```python
from build123d import *

# Parameters (mm, degrees)
BOSS_EXTRUDE1_DEPTH = 12
SKETCH3_R           = 2
CUT_EXTRUDE1_DEPTH  = 10
SKETCH4_R           = 3
CUT_EXTRUDE2_DEPTH  = 10


with BuildPart() as part:
    # Sketch2 → Boss-Extrude1 (new body)
    with BuildSketch(Plane.XY):
        with BuildLine():
            Line((-25, 0), (-12.5, 0))
            ThreePointArc((-12.5, 0), (0, 12.5), (12.5, 0))
            Line((12.5, 0), (25, 0))
            ThreePointArc((25, 0), (24.873403825, 2.51272405), (24.494897428, 5))
            Line((24.494897428, 5), (21.563858653, 5))
            ThreePointArc((21.563858653, 5), (19.850737931, 5.537233793), (18.751181437, 6.956521739))
            ThreePointArc((18.751181437, 6.956521739), (0, 20), (-18.751181437, 6.956521739))
            ThreePointArc((-18.751181437, 6.956521739), (-19.850737931, 5.537233793), (-21.563858653, 5))
            Line((-21.563858653, 5), (-24.494897428, 5))
            ThreePointArc((-24.494897428, 5), (-24.873403825, 2.51272405), (-25, 0))
        make_face()
    extrude(amount=BOSS_EXTRUDE1_DEPTH)

    # Sketch3 → Cut-Extrude1 (cut)
    with BuildSketch(Plane(origin=(0, 0, 0), x_dir=(1, 0, 0), z_dir=(0, 1, 0))):
        with Locations(Location((20, -6, 0), (0, 0, 128.638810709))):
            Circle(SKETCH3_R)
        with Locations(Location((-20, -6, 0), (0, 0, 90))):
            Circle(SKETCH3_R)
    extrude(amount=CUT_EXTRUDE1_DEPTH, mode=Mode.SUBTRACT)

    # Sketch4 → Cut-Extrude2 (cut)
    with BuildSketch(Plane(origin=(0, 5, 0), x_dir=(1, 0, 0), z_dir=(0, 1, 0))):
        with Locations((20, -6)):
            Circle(SKETCH4_R)
        with Locations((-20, -6)):
            Circle(SKETCH4_R)
    extrude(amount=CUT_EXTRUDE2_DEPTH, mode=Mode.SUBTRACT)


solid = part.part
```
Input: part model. Units: mm. Frame: model coordinates. Give positions to 0.01 mm unless a question says otherwise; leave off trailing zeros. Order: outer loops, then holes, each group sorted by start corner. A loop starts at its lowest first (then second) coordinate and runs counter-clockwise, first axis right, second up. Notation, with made-up numbers: (-28.5, 33.5) - (28.5, 33.5) arc R5 cw to (28.5, 41.5) - close; hole circle Ø6 at (-22, -38). An arc over 180 degrees is marked (long way). Put each result on its own line as item: value.
Item 1: Section query A-A, the plane z = 6. Return loops of the section in (x, y), then the cut area to 3 significant figures.
Found:
outline: (-25, 0) - (-22, 0) - (-22, 5) - (-24.49, 5) arc R25 ccw to start; (-18, 0) - (-12.5, 0) arc R12.5 cw to (12.5, 0) - (18, 0) - (18, 5) - (17, 5) - (17, 10.54) arc R20 ccw to (-17, 10.54) - (-17, 5) - (-18, 5) - close; (22, 0) - (25, 0) arc R25 ccw to (24.49, 5) - (22, 5) - close
area: 378 mm^2
Item 2: Section query B-B, the plane x = -20. Return loops of the section in (y, z), then the cut area to 3 significant figures.
Found:
outline: (0, 0) - (5.44, 0) - (5.44, 3) - (5, 3) - (5, 4) - (0, 4) - close; (0, 8) - (5, 8) - (5, 9) - (5.44, 9) - (5.44, 12) - (0, 12) - close
area: 42.6 mm^2
Item 3: Draft query along X for faces 1 (the cylindrical face through (-22, 2, 6)), 2 (the flat face through (0, 15, 0)), 3 (the cylindrical face through (-19.83, 5.55, 1.7)). Return one class per face: +X half, -X half, draft (parallel to the pull), parting line (faces both ways), or undercut.
Found:
face 1: undercut
face 2: draft
face 3: -X half
Item 4: Section query D-D, the plane x = 0. Return loops of the section in (y, z).
Found:
outline: (12.5, 0) - (20, 0) - (20, 12) - (12.5, 12) - close
Item 5: Contact query for flat-ended pins moving along their axis: pin 1 (3 mm diameter, centred on x = -12.5, y = 8, fed in from -Z); pin 2 (5 mm diameter, centred on y = 8.5, z = 9, fed in from -X); pin 3 (2 mm diameter, centred on x = -20, z = 7.5, fed in from +Y); pin 4 (6 mm diameter, centred on x = 19, z = 5, fed in from +Y). Output: stop coordinate, or through.
Found:
pin 1: stops at z = 0
pin 2: stops at x = -19.33
pin 3: stops at y = 5
pin 4: stops at y = 12
Item 6: Ray query, L1, parallel to X at y = 3.4, z = 6; L2, parallel to X at y = 2.3, z = 6; L3, parallel to Z at x = 20, y = 3.5. Return the intervals inside material, ascending. Write a range as from..to.
Found:
L1: x = -24.77..-22, -18..-12.03, 12.03..18, 22..24.77
L2: x = -24.89..-22, -18..-12.29, 12.29..18, 22..24.89
L3: z = 0..4, 8..12
Item 7: Section query C-C, the plane y = 5.5. Return loops of the section in (x, z).
Found:
outline: (-19.91, 0) - (-11.22, 0) - (-11.22, 12) - (-19.91, 12) - (-19.91, 9) arc R3 cw to (-19.91, 3) - close; (11.22, 0) - (19.91, 0) - (19.91, 3) arc R3 cw to (19.91, 9) - (19.91, 12) - (11.22, 12) - close
